from build123d import *

# Parameters (mm, degrees)
CROQUIS1_W              = 20
CROQUIS1_H              = 40
SALIENTE_EXTRUIR1_DEPTH = 10
CROQUIS5_R              = 6.7
CORTAR_EXTRUIR1_DEPTH   = 40
CROQUIS6_W              = 40
CROQUIS6_H              = 15
SALIENTE_EXTRUIR2_DEPTH = 10
CROQUIS7_W              = 7
CROQUIS7_H              = 40
CORTAR_EXTRUIR2_DEPTH   = 15
CROQUIS8_R              = 1.7
CORTAR_EXTRUIR3_DEPTH   = 20
REDONDEO1_R             = 4
REDONDEO2_R             = 5


with BuildPart() as part:
    # Croquis1 → Saliente-Extruir1 (new body, symmetric)
    with BuildSketch(Plane(origin=(0, 0, 0), x_dir=(1, 0, 0), z_dir=(0, 1, 0))):
        Rectangle(CROQUIS1_W, CROQUIS1_H)
    extrude(amount=SALIENTE_EXTRUIR1_DEPTH, both=True)

    # Croquis5 → Cortar-Extruir1 (cut)
    with BuildSketch(Plane(origin=(0, 0, -20), x_dir=(-1, 0, 0), z_dir=(0, 0, -1))):
        Circle(CROQUIS5_R)
    extrude(amount=-CORTAR_EXTRUIR1_DEPTH, mode=Mode.SUBTRACT)

    # Croquis6 → Saliente-Extruir2 (add, symmetric)
    with BuildSketch(Plane(origin=(0, 0, 0), x_dir=(0, 0, -1), z_dir=(1, 0, 0))):
        with Locations((20, 17.5)):
            Rectangle(CROQUIS6_W, CROQUIS6_H)
    extrude(amount=SALIENTE_EXTRUIR2_DEPTH, both=True)

    # Croquis7 → Cortar-Extruir2 (cut)
    with BuildSketch(Plane(origin=(0, 25, 0), x_dir=(1, 0, 0), z_dir=(0, 1, 0))):
        with Locations((0, 20)):
            Rectangle(CROQUIS7_W, CROQUIS7_H)
    extrude(amount=-CORTAR_EXTRUIR2_DEPTH, mode=Mode.SUBTRACT)

    # Croquis8 → Cortar-Extruir3 (cut)
    with BuildSketch(Plane(origin=(10, 0, 0), x_dir=(0, 0, -1), z_dir=(1, 0, 0))):
        with Locations((6, 17.5)):
            Circle(CROQUIS8_R)
        with Locations((34, 17.5)):
            Circle(CROQUIS8_R)
    extrude(amount=-CORTAR_EXTRUIR3_DEPTH, mode=Mode.SUBTRACT)

    # Redondeo1
    redondeo1_edges = [part.edges().sort_by_distance(p)[0] for p in [
        (6.75, 10, -40),
        (6.75, 25, -40),
        (6.75, 25, 0),
        (-6.75, 25, 0),
        (-6.75, 25, -40),
        (-6.75, 10, -40),
        (-6.75, 10, -20),
        (6.75, 10, -20),
    ]]
    fillet(redondeo1_edges, radius=REDONDEO1_R)

    # Redondeo2
    redondeo2_edges = [part.edges().sort_by_distance(p)[0] for p in [
        (-10, 10, 10),
        (10, 10, 10),
        (-10, -10, 0),
        (10, -10, 0),
    ]]
    fillet(redondeo2_edges, radius=REDONDEO2_R)


solid = part.part
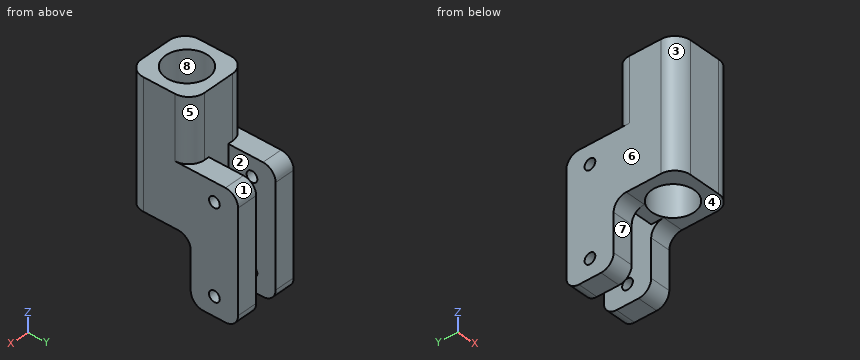
Design review of the part built by this model. Coordinates are the model's own, in mm. Face numbers are marked on the shaded views. A direction names the side the tool comes from. Give positions to 0.01 mm unless a question says otherwise; leave off trailing zeros. Order: outer loops, then holes, each group sorted by start corner. A loop starts at its lowest first (then second) coordinate and runs counter-clockwise, first axis right, second up. Notation, with made-up numbers: (7, 24.5) - (53, 24.5) arc R12 ccw to (53, 46.5) - close; hole circle Ø8 at (22, 49.25). An arc over 180 degrees is marked (long way). Write item = value, one per line. Start each with the question number.
Q1. To check wall thickness, follow L1, parallel to X at y = 23.5, z = -6.5; L2, parallel to X at y = 3, z = -11.5; L3, parallel to Y at x = 0, z = 7. State the ranges of each line that lie inside material, in increasing order. Write a range as from..to.
Q2. We need section D-D on z = -34. State the section outline as (x, y) points.
Q3. Mouldability with a two-part tool opening along X and no side actions: class the marked faces 1, 2 and 3 as released by +X, released by -X, zero draft, split by the parting line, or undercut.
Q4. Clearance check with flat-ended pins moving along their axes: pin 1 Ø8 at (x, y) = (8, -3) entering from -Z; pin 2 Ø3 at (x, y) = (8.5, 17) entering from +Z; pin 3 Ø2 at (x, y) = (-4, 12.5) entering from -Z. State where each tip first meets the part, or that it passes through.
Q5. We need section A-A on y = 17.5. State the section outline as (x, z) points, plus the area to 3 significant figures.
Q6. We need section C-C on x = 0. State the section outline as (y, z) points.
Q7. Tool access review of the marked faces 4, 5, 6, 7 and 8: name each direction out of +Z, -Z, +X, -X, +Y, -Y from which nothing blocks a thin tool from reaching the whole face with its end or side.
Q8. We need section B-B on z = -6. State the section outline as (x, y) points, plus the area to 3 significant figures.
Working result:
q1.L1 = -10..-3.5, 3.5..10
q1.L2 = -10..-5.99, 5.99..10
q1.L3 = -10..-6.7, 6.7..10
q2.outline = (-10, 10) - (-3.5, 10) - (-3.5, 15.8) - (-10, 15.8) - close; (-10, 19.2) - (-3.5, 19.2) - (-3.5, 25) - (-10, 25) - close; (3.5, 10) - (10, 10) - (10, 15.8) - (3.5, 15.8) - close; (3.5, 19.2) - (10, 19.2) - (10, 25) - (3.5, 25) - close
q3.face_1 = zero draft
q3.face_2 = undercut
q3.face_3 = released by -X
q4.pin_1 = -20
q4.pin_2 = 0
q4.pin_3 = -39.97
q5.outline = (-10, -40) - (-3.5, -40) - (-3.5, -35.7) - (-10, -35.7) - close; (-10, -32.3) - (-3.5, -32.3) - (-3.5, -7.7) - (-10, -7.7) - close; (-10, -4.3) - (-3.5, -4.3) - (-3.5, 0) - (-10, 0) - close; (3.5, -40) - (10, -40) - (10, -35.7) - (3.5, -35.7) - close; (3.5, -32.3) - (10, -32.3) - (10, -7.7) - (3.5, -7.7) - close; (3.5, -4.3) - (10, -4.3) - (10, 0) - (3.5, 0) - close
q5.area = 432 mm²
q6.outline = (-10, -20) - (-6.7, -20) - (-6.7, 20) - (-10, 20) - close; (6.7, -20) - (10, -20) - (10, 20) - (6.7, 20) - close
q7.face_4 = -Z, -Y
q7.face_5 = +Z, +X, +Y
q7.face_6 = +Z, -Z, -X, +Y, -Y
q7.face_7 = -Z, +X, -X, -Y
q7.face_8 = +Z, -Z
q8.outline = (-10, -5) arc R5 ccw to (-5, -10) - (5, -10) arc R5 ccw to (10, -5) - (10, 15.8) - (3.5, 15.8) - (3.5, 10) - (-3.5, 10) - (-3.5, 15.8) - (-10, 15.8) - close; (-10, 19.2) - (-3.5, 19.2) - (-3.5, 25) - (-10, 25) - close; (3.5, 19.2) - (10, 19.2) - (10, 25) - (3.5, 25) - close; hole circle Ø13.4 at (0, 0)
q8.area = 399 mm²
